The figure shows three views and two pictorial views of one solid part (mm, origin at its lowest corner). Answer the questions. A direction names the side the tool comes from. Coordinates: 2 decimals unless noted, no trailing zeros. Loops run counter-clockwise (first coordinate to the right, second up) from the corner with the lowest first, then second, coordinate; pieces in that order, holes last. Notation, with made-up numbers: (68, 39.25) -> (92, 39.25) arc R31 ccw to (92, 69.25) -> close; hole circle Ø8 at (-34, 42). An arc over 180 degrees is marked (long way). Answer as a JSON object with one key per item and string values. Group by question number.
1) Section C-C, the plane z = 25 is taken. Give the vertices of the cut face in (x, y).
2) Section D-D, the plane x = 25 is taken. Give the vertices of the cut face in (y, z), plus the area to 3 significant figures.
3) Consider probe 1 along Y at (x, z) = (0.8, 25); probe 2 along Z at (x, y) = (16, 41.5). Determine where each line is inside the solid, lowest interval first. Write a range as [from, to].
4) Flat-ended cylindrical pins translate along their axes: P1, Ø4, axis at y = 20.5, z = 12, coming from the -X side; P2, Ø13.5, axis at x = 25, y = 55, coming from the +Z side; P3, Ø8.5, axis at y = 55, z = 25, coming from the -X side. Find the tip coordinate at first contact, or state that the pin passes through.
5) Determine the mould class of the marked faces 1, 2 and 3 for opening direction X: released by +X, released by -X, zero draft, split by the parting line, or undercut.
6) Section A-A, the plane y = 55 is taken. Count the separate pieces of the cut face and the enclosed holes in it, plus the area to 3 significant figures.
7) Section B-B, the plane x = 6.5 is taken. Give the vertices of the cut face in (y, z), plus the area to 3 significant figures.
8) Which of the six approach directions +Z, -Z, +X, -X, +Y, -Y give full straight-line access (tool end or side, diameter ignored) to the marked faces 4 and 5?
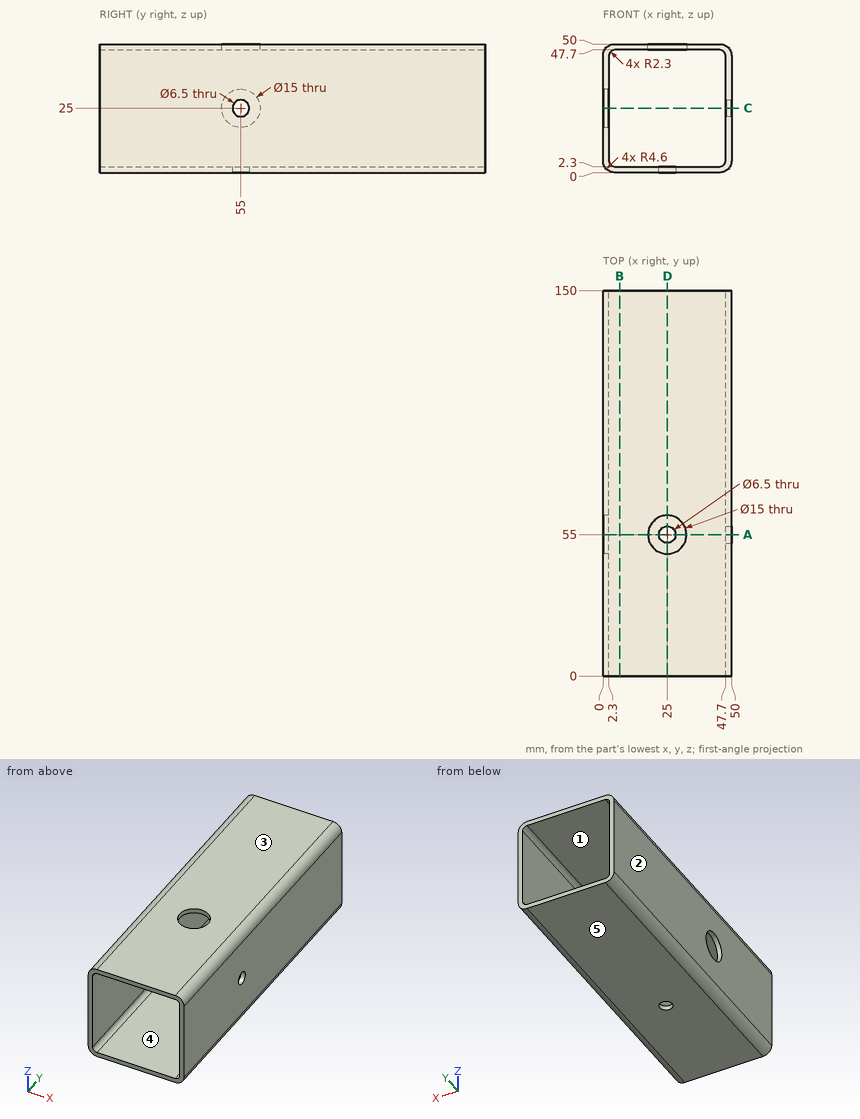
Determined:
{
 "1": {"outline": "(0, 0) -> (2.3, 0) -> (2.3, 47.5) -> (0, 47.5) -> close; (0, 62.5) -> (2.3, 62.5) -> (2.3, 150) -> (0, 150) -> close; (47.7, 0) -> (50, 0) -> (50, 51.75) -> (47.7, 51.75) -> close; (47.7, 58.25) -> (50, 58.25) -> (50, 150) -> (47.7, 150) -> close"},
 "2": {"outline": "(0, 0) -> (51.75, 0) -> (51.75, 2.3) -> (0, 2.3) -> close; (0, 47.7) -> (47.5, 47.7) -> (47.5, 50) -> (0, 50) -> close; (58.25, 0) -> (150, 0) -> (150, 2.3) -> (58.25, 2.3) -> close; (62.5, 47.7) -> (150, 47.7) -> (150, 50) -> (62.5, 50) -> close", "area": "641 mm²"},
 "3": {"probe 1": "[0, 47.5], [62.5, 150]", "probe 2": "[0, 2.3], [47.7, 50]"},
 "4": {"P1": "x = 0", "P2": "z = 2.3", "P3": "x = 47.7"},
 "5": {"face 1": "undercut", "face 2": "released by -X", "face 3": "zero draft"},
 "6": {"separate pieces": "4", "enclosed holes": "0", "area": "326 mm²"},
 "7": {"outline": "(0, 0) -> (150, 0) -> (150, 2.3) -> (0, 2.3) -> close; (0, 47.7) -> (150, 47.7) -> (150, 50) -> (0, 50) -> close", "area": "690 mm²"},
 "8": {"face 4": "+Y, -Y", "face 5": "-Z, +X, -X, +Y, -Y"}
}
